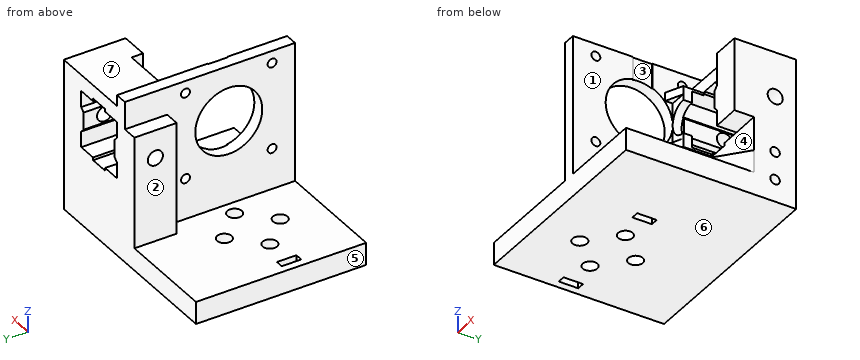
from build123d import *

# Parameters (mm, degrees)
SKETCH007_W         = 74.914368
SKETCH007_H         = 60.949894
SKETCH007_R         = 2.6
SKETCH007_W_2       = 2.75
SKETCH007_H_2       = 7
PAD005_DEPTH        = 8
SKETCH009_W         = 40
SKETCH009_H         = 15.144356
PAD006_DEPTH        = 40.1
POCKET004_DEPTH     = 50
PAD007_DEPTH        = 50
PAD008_DEPTH        = 7
PAD009_DEPTH        = 7
SKETCH012_R         = 2.7
POCKET005_DEPTH     = 1000
SKETCH014_R         = 12
SKETCH014_R_2       = 1.6
POCKET006_DEPTH     = 5
SKETCH015_W         = 30.1
SKETCH015_H         = 16
PAD010_DEPTH        = 21.5
PAD010_TAPER        = 20
PAD010_FACE47_W     = 4.5
PAD010_FACE47_H     = 9.9
PAD011_DEPTH        = 16
PAD011_FACE21_W     = 0.855644
PAD011_FACE21_H     = 4.5
POCKET007_DEPTH     = 20
SKETCH016_R         = 1.7
POCKET008_DEPTH     = 18
LINEARPATTERN_COUNT = 2
LINEARPATTERN_PITCH = 10
PAD015_DEPTH        = 6
PAD016_DEPTH        = 3
PAD017_DEPTH        = 3
SKETCH027_R         = 6
POCKET010_DEPTH     = 3.2
POCKET010_FACE26_W  = 22.144356
POCKET010_FACE26_H  = 9.9
PAD018_DEPTH        = 6
PAD_DEPTH           = 18
SKETCH_W            = 6
SKETCH_H            = 0.836678
PAD019_DEPTH        = 7
SKETCH029_W         = 6
SKETCH029_H         = 0.8
PAD020_DEPTH        = 10


with BuildPart() as part:
    # Sketch007 → Pad005 (new body)
    with BuildSketch(Plane.XY):
        with Locations((12.457184, 5.474947)):
            Rectangle(SKETCH007_W, SKETCH007_H)
        with Locations((0, 10)):
            Circle(SKETCH007_R, mode=Mode.SUBTRACT)
        with Locations((10, 0)):
            Circle(SKETCH007_R, mode=Mode.SUBTRACT)
        with Locations((-10, 0)):
            Circle(SKETCH007_R, mode=Mode.SUBTRACT)
        with Locations((0, -10)):
            Circle(SKETCH007_R, mode=Mode.SUBTRACT)
        with Locations((20.875, 0)):
            Rectangle(SKETCH007_W_2, SKETCH007_H_2, mode=Mode.SUBTRACT)
        with Locations((-20.875, 0)):
            Rectangle(SKETCH007_W_2, SKETCH007_H_2, mode=Mode.SUBTRACT)
    extrude(amount=PAD005_DEPTH)

    # Sketch009 (on Face18 of Pad005) → Pad006 (join)
    with BuildSketch(Plane.XY.offset(8)):
        with Locations((29.914368, 28.377716)):
            Rectangle(SKETCH009_W, SKETCH009_H)
    extrude(amount=PAD006_DEPTH)

    # Sketch010 (on Face19 of Pad006) → Pocket004 (cut)
    with BuildSketch(Plane.XZ.offset(-20.805538)):
        Polygon((19.814368, 48.1), (19.814368, 42.426645), (21.140392, 41.059428), (21.140392, 34.859428), (19.814368, 33.573355), (19.814368, 27.9), (26.496015, 27.9), (26.496015, 26.9), (33.332721, 26.9), (33.332721, 27.9), (40.014368, 27.9), (40.014368, 33.573355), (38.689334, 34.965349), (38.689334, 41.165349), (40.014368, 42.426645), (40.014368, 48.1), align=None)
    extrude(amount=-POCKET004_DEPTH, mode=Mode.SUBTRACT)

    # Sketch011 (on Face5 of Pocket004) → Pad007 (join)
    with BuildSketch(Plane.XY.offset(8)):
        Polygon((15.314368, 20.805538), (15.314368, -25), (19.814368, -25), (19.814368, -3.5), (19.5, -3.5), (19.5, 3.5), (19.814368, 3.5), (19.814368, 20.805538), align=None)
    extrude(amount=PAD007_DEPTH)

    # Sketch013 (on Face34 of Pad007) → Pad008 (join)
    with BuildSketch(Plane.XZ.offset(-20.805538)):
        Polygon((40.014368, 48.1), (40.014368, 42.426645), (38.689334, 41.165349), (38.689334, 34.965349), (40.014368, 33.573355), (40.014368, 27.9), (49.914368, 28.05), (49.914368, 48.1), align=None)
    extrude(amount=PAD008_DEPTH)

    # Pad008 Face35 → Pad009 (add)
    with BuildSketch(Plane(origin=(20.438426, 20.805538, 37.980906), x_dir=(-1, 0, 0), z_dir=(0, -1, 0))):
        Polygon((0.624058, 4.407551), (-0.701966, 3.121478), (-0.701966, -3.078522), (0.624058, -4.445739), align=None)
    extrude(amount=PAD009_DEPTH)

    # Sketch012 (on Face5 of Pad007) → Pocket005 (cut)
    with BuildSketch(Plane.YZ.offset(49.914368)):
        with Locations((28.429679, 38.1)):
            Circle(SKETCH012_R)
    extrude(amount=-POCKET005_DEPTH, mode=Mode.SUBTRACT)

    # Sketch014 (on Face25 of Pocket005) → Pocket006 (cut)
    with BuildSketch(Plane.YZ.offset(19.814368)):
        with Locations((-1.267852, 38.1)):
            Circle(SKETCH014_R)
        with Locations((-16.767852, 53.6)):
            Circle(SKETCH014_R_2)
        with Locations((14.232148, 53.6)):
            Circle(SKETCH014_R_2)
        with Locations((14.232148, 22.6)):
            Circle(SKETCH014_R_2)
        with Locations((-16.767852, 22.6)):
            Circle(SKETCH014_R_2)
    extrude(amount=-POCKET006_DEPTH, mode=Mode.SUBTRACT)

    # Sketch015 (on Face41 of Pocket006) → Pad010 (join)
    with BuildSketch(Plane.XZ.offset(-20.805538)):
        with Locations((34.864368, 8)):
            Rectangle(SKETCH015_W, SKETCH015_H)
    extrude(amount=PAD010_DEPTH, taper=PAD010_TAPER)

    # Pad010 Face47 → Pad011 (add)
    with BuildSketch(Plane(origin=(17.564368, 20.805538, 53.05), x_dir=(1, 0, 0), z_dir=(0, 1, 0))):
        Rectangle(PAD010_FACE47_W, PAD010_FACE47_H)
    extrude(amount=PAD011_DEPTH)

    # Pad011 Face21 → Pocket007 (cut)
    with BuildSketch(Plane(origin=(17.564368, 36.377716, 48.1), x_dir=(0, -1, 0), z_dir=(0, 0, -1))):
        Rectangle(PAD011_FACE21_W, PAD011_FACE21_H)
    extrude(amount=-POCKET007_DEPTH, mode=Mode.SUBTRACT)

    # Sketch016 (on Face5 of Pocket007) → Pocket008 (cut)
    with BuildSketch(Plane.YZ.offset(49.914368)):
        with Locations((28.377716, 8)):
            Circle(SKETCH016_R)
    pocket008 = extrude(amount=-POCKET008_DEPTH, mode=Mode.SUBTRACT)

    # LinearPattern: Pocket008 ×2
    with Locations(*[(0, 0, i * LINEARPATTERN_PITCH) for i in range(1, LINEARPATTERN_COUNT)]):
        add(pocket008, mode=Mode.SUBTRACT)

    # Sketch021 (on Face11 of LinearPattern) → Pad015 (join)
    with BuildSketch(Plane.YZ.offset(19.814368)):
        Polygon((10.732148, 38.1), (10.732148, 49.1), (13.805538, 49.1), (13.805538, 27.1), (10.732148, 27.1), align=None)
    extrude(amount=PAD015_DEPTH)

    # Sketch025 (on Face62 of Pad015) → Pad016 (join)
    with BuildSketch(Plane(origin=(0, 0, 27.1), x_dir=(1, 0, 0), z_dir=(0, 0, -1))):
        Polygon((25.814368, -10.732148), (19.814368, -10.732148), (19.814368, -8.062612), align=None)
    extrude(amount=-PAD016_DEPTH)

    # Sketch026 (on Face59 of Pad016) → Pad017 (join)
    with BuildSketch(Plane.XY.offset(49.1)):
        Polygon((19.814368, 10.732148), (25.814368, 10.732148), (19.814368, 8.062148), align=None)
    extrude(amount=-PAD017_DEPTH)

    # Sketch027 (on Face61 of Pad017) → Pocket010 (cut)
    with BuildSketch(Plane.XZ.offset(-10.732148)):
        with Locations((25.814368, 38.1)):
            Circle(SKETCH027_R)
    extrude(amount=-POCKET010_DEPTH, mode=Mode.SUBTRACT)

    # Pocket010 Face26 → Pad018 (add)
    with BuildSketch(Plane(origin=(44.964368, 24.877716, 48.1), x_dir=(0, 1, 0), z_dir=(0, 0, 1))):
        Rectangle(POCKET010_FACE26_W, POCKET010_FACE26_H)
    extrude(amount=PAD018_DEPTH)

    # Sketch028 (on Face68 of Pad018) → Pad (join)
    with BuildSketch(Plane(origin=(0, 35.949894, 0), x_dir=(-1, 0, 0), z_dir=(0, 1, 0))):
        Polygon((-40.014368, 48.263322), (-33.332721, 48.263322), (-33.332721, 49.263322), (-26.496015, 49.263322), (-26.496015, 48.263322), (-19.814368, 48.263322), (-19.814368, 54.1), (-40.014368, 54.1), align=None)
    extrude(amount=-PAD_DEPTH)

    # Sketch (on Face49 of Pad) → Pad019 (join)
    with BuildSketch(Plane.XZ.offset(-17.949894)):
        with Locations((22.814368, 48.681661)):
            Rectangle(SKETCH_W, SKETCH_H)
    extrude(amount=PAD019_DEPTH)

    # Sketch029 (on Face63 of Pad019) → Pad020 (join)
    with BuildSketch(Plane.XZ.offset(-20.805538)):
        with Locations((22.814368, 27.5)):
            Rectangle(SKETCH029_W, SKETCH029_H)
    extrude(amount=PAD020_DEPTH)


solid = part.part
The model under review builds one solid part; all positions refer to its coordinate system, in mm. Face numbers are marked on the shaded views. A direction names the side the tool comes from. Coordinates: 2 decimals unless noted, no trailing zeros. Write each loop counter-clockwise with the first axis right and the second up, starting at its lowest first coordinate (ties: lowest second). Pieces come first, ordered by that corner, then holes. Notation, with made-up numbers: (33.25, 84.5) - (60.25, 84.5) arc R11 ccw to (60.25, 95.5) - close; hole circle Ø1 at (-7.5, -14.5). An arc over 180 degrees is marked (long way). Answer as a JSON object with one key per item and string values. Group by question number.
1. Mouldability with a two-part tool opening along Z and no side actions: class the marked faces 4, 5, 6 and 7 as pulls with the +Z half, pulls with the -Z half, needs draft (parallel to the pull), parting line crosses it, or undercut.
2. Machinability: for the marked faces 1, 2 and 3, which of the approach directions +Z, -Z, +X, -X, +Y, -Y give a long, thin tool a straight path to every point of the face, cutting with its end or side? Answer none if there is none.
3. Clearance check with flat-ended pins moving along their axes: pin 1 Ø6 at (y, z) = (-12, 45) entering from -X; pin 2 Ø10 at (x, z) = (3.5, 14) entering from -Y; pin 3 Ø5 at (x, y) = (3.5, 29) entering from +Z; pin 4 Ø1.8 at (x, z) = (31, 50) entering from -Y. State where each tip first meets the part, or that it passes through.
4. To check wall thickness, follow probe 1 along Z at (x, y) = (35.5, 33); probe 2 along X at (y, z) = (17.5, 49); probe 3 along X at (y, z) = (13, 14.5). State the ranges of each line that lie inside material, in increasing order.
5. Add section D-D (x = 9). Give the boundary of the cut face in (y, z).
6. Add section C-C (x = 0). Give the boundary of the cut face in (y, z).
7. Add section A-A (x = -10). Give the boundary of the cut face in (y, z).
8. Add section B-B (y = -10). Give the boundary of the cut face in (x, z).
Findings:
{
 "1": {"face 4": "undercut", "face 5": "needs draft", "face 6": "pulls with the -Z half", "face 7": "pulls with the +Z half"},
 "2": {"face 1": "+Z, +X, -Y", "face 2": "+Z, -X, +Y, -Y", "face 3": "+Z, -Z, +X"},
 "3": {"pin 1": "x = 15.31", "pin 2": "through", "pin 3": "z = 8", "pin 4": "y = 17.95"},
 "4": {"probe 1": "0 to 27.9, 48.26 to 54.1", "probe 2": "15.31 to 25.81, 40.01 to 49.91", "probe 3": "15.31 to 19.81"},
 "5": {"outline": "(-25, 0) - (-2.4, 0) - (-2.4, 8) - (-25, 8) - close; (2.4, 0) - (35.95, 0) - (35.95, 8) - (2.4, 8) - close"},
 "6": {"outline": "(-25, 0) - (-12.6, 0) - (-12.6, 8) - (-25, 8) - close; (-7.4, 0) - (7.4, 0) - (7.4, 8) - (-7.4, 8) - close; (12.6, 0) - (35.95, 0) - (35.95, 8) - (12.6, 8) - close"},
 "7": {"outline": "(-25, 0) - (-2.6, 0) - (-2.6, 8) - (-25, 8) - close; (2.6, 0) - (35.95, 0) - (35.95, 8) - (2.6, 8) - close"},
 "8": {"outline": "(-25, 0) - (-2.6, 0) - (-2.6, 8) - (-25, 8) - close; (2.6, 0) - (49.91, 0) - (49.91, 8) - (19.81, 8) - (19.81, 29.87) - (15.31, 29.87) - (15.31, 8) - (2.6, 8) - close; (15.31, 46.33) - (19.81, 46.33) - (19.81, 58) - (15.31, 58) - close"}
}
